from build123d import *

# Parameters (mm, degrees)
SKETCH1_R                 = 4.7625
BOSS_EXTRUDE1_DEPTH       = 6.604
CUT_EXTRUDE1_DEPTH        = 7.604
SKETCH3_W                 = 6.604
SKETCH3_H                 = 6.35
BOSS_EXTRUDE2_DEPTH       = 6.604
FILLET1_R                 = 6.35
FILLET2_R                 = 3.175
F_4_40_TAPPED_HOLE1_D     = 2.2606
F_4_40_TAPPED_HOLE1_DEPTH = 7.5946
F_4_40_TAPPED_HOLE1_TIP   = 0.679152758


with BuildPart() as part:
    # Sketch1 → Boss-Extrude1 (new body)
    with BuildSketch(Plane.XY):
        Polygon((0, 0), (0, 69.85), (-19.939, 69.85), (-19.939, 50.8), (-25.4, 45.339), (-25.4, 0), align=None)
        with Locations((-9.9695, 57.15)):
            Circle(SKETCH1_R, mode=Mode.SUBTRACT)
    extrude(amount=BOSS_EXTRUDE1_DEPTH)

    # Sketch2 → Cut-Extrude1 (cut, through all)
    with BuildSketch(Plane.XY.offset(6.604)):
        Polygon((-12.2936, 37.0078), (-13.716, 37.0078), (-13.716, 32.8422), (-12.2936, 32.8422), (-12.2936, 30.5562), (-6.35, 30.5562), (-6.35, 32.8422), (0, 32.8422), (0, 37.0078), (-6.35, 37.0078), (-6.35, 39.2938), (-12.2936, 39.2938), align=None)
        Polygon((-12.2936, 20.2438), (-12.2936, 17.9578), (-13.716, 17.9578), (-13.716, 13.7922), (-12.2936, 13.7922), (-12.2936, 11.5062), (-6.35, 11.5062), (-6.35, 13.7922), (0, 13.7922), (0, 17.9578), (-6.35, 17.9578), (-6.35, 20.2438), align=None)
    extrude(amount=-CUT_EXTRUDE1_DEPTH, mode=Mode.SUBTRACT)

    # Sketch3 → Boss-Extrude2 (add)
    with BuildSketch(Plane.XY.offset(6.604)):
        with Locations((3.302, 44.45)):
            Rectangle(SKETCH3_W, SKETCH3_H)
        with Locations((3.302, 25.4)):
            Rectangle(SKETCH3_W, SKETCH3_H)
        with Locations((3.302, 6.35)):
            Rectangle(SKETCH3_W, SKETCH3_H)
    extrude(amount=-BOSS_EXTRUDE2_DEPTH)

    # Fillet1
    fillet1_edges = [part.edges().sort_by_distance(p)[0] for p in [
        (-25.4, 0, 3.302),
        (-25.4, 45.339, 3.302),
        (-19.939, 50.8, 3.302),
        (0, 69.85, 3.302),
    ]]
    fillet(fillet1_edges, radius=FILLET1_R)

    # Fillet2
    fillet2_edges = [part.edges().sort_by_distance(p)[0] for p in [
        (-19.939, 69.85, 3.302),
    ]]
    fillet(fillet2_edges, radius=FILLET2_R)

    # #4-40 Tapped Hole1
    with Locations(Plane.XY.offset(6.604)):
        with Locations((-3.6195, 49.53), (-16.3195, 49.53)):
            Hole(F_4_40_TAPPED_HOLE1_D / 2, depth=F_4_40_TAPPED_HOLE1_DEPTH)
            with Locations((0, 0, -(F_4_40_TAPPED_HOLE1_DEPTH + F_4_40_TAPPED_HOLE1_TIP / 2))):  # 118° drill point
                Cone(0, F_4_40_TAPPED_HOLE1_D / 2, F_4_40_TAPPED_HOLE1_TIP, mode=Mode.SUBTRACT)


solid = part.part
For this review, take the finished solid that the model builds, in its own axes (mm). A direction names the side the tool comes from. Give positions to 0.01 mm unless a question says otherwise; leave off trailing zeros. Order: outer loops, then holes, each group sorted by start corner. A loop starts at its lowest first (then second) coordinate and runs counter-clockwise, first axis right, second up. Notation, with made-up numbers: M 48.25,-36.75 L 98.25,-36.75 A19 cw 98.25,-31.75 Z; hole C -5.75,81 d2. An arc over 180 degrees is marked long. Answer in a Markdown table with one row per item. Add a question column.
(1) For pin 1 (4 mm diameter, centred on x = -8, y = 7, fed in from -Z); pin 2 (1.1 mm diameter, centred on y = 12.5, z = 2, fed in from +X); pin 3 (3.5 mm diameter, centred on x = 3.5, z = 4, fed in from +Y) (3 decimals); pin 4 (2 mm diameter, centred on x = -10, y = 55, fed in from +Z), all flat-tipped, find the tip position at first contact; note any pin that passes through.
(2) Mouldability with a two-part tool opening along Y and no side actions: class faces 1 (the face through (-3, 32.842, 3)), 2 (the face through (6.604, 6, 3)), 3 (the face through (-1.91, 68.04, 3.35)) as +Y half, -Y half, draft (parallel to the pull), parting line (faces both ways), or undercut.
(3) Consider section B-B on x = -8. State the section outline as (y, z) points, and give its area (3 significant figures).
(4) Consider section A-A on y = 57.15. State the section outline as (x, z) points, and give its area (3 significant figures).
(5) Consider section C-C on z = 0.75. Give the number of separate pieces and of enclosed holes in the cut face, and give its area (3 significant figures).
(6) Wall thickness on probe 1 along Y at (x, z) = (-6.5, 6.25); probe 2 along Y at (x, z) = (-7, 4); probe 3 along X at (y, z) = (18, 4.5): over which ranges is each line inside the solid? List them lowest first. Write a range as [from, to].
(7) For faces 4 (the face through (0, 2, 3)), 5 (the face through (-9, 11.506, 3)), 6 (the face through (-13, 17.958, 3)), list the 3-axis set-ups (+Z, -Z, +X, -X, +Y, -Y) from which the entire face can be reached by the end or side of a thin tool; tool diameter is ignored.
Evaluation:
| question | item | result |
|---|---|---|
| 1 | pin 1 | stops at z = 0 |
| 1 | pin 2 | stops at x = 0 |
| 1 | pin 3 | stops at y = 47.625 |
| 1 | pin 4 | passes through |
| 2 | face 1 | undercut |
| 2 | face 2 | draft |
| 2 | face 3 | +Y half |
| 3 | outline | M 0,0 L 11.51,0 L 11.51,6.6 L 0,6.6 Z; M 20.24,0 L 30.56,0 L 30.56,6.6 L 20.24,6.6 Z; M 39.29,0 L 52.81,0 L 52.81,6.6 L 39.29,6.6 Z; M 61.49,0 L 69.85,0 L 69.85,6.6 L 61.49,6.6 Z |
| 3 | area | 289 mm^2 |
| 4 | outline | M -19.94,0 L -14.73,0 L -14.73,6.6 L -19.94,6.6 Z; M -5.21,0 L 0,0 L 0,6.6 L -5.21,6.6 Z |
| 4 | area | 68.8 mm^2 |
| 5 | separate pieces | 1 |
| 5 | enclosed holes | 3 |
| 5 | area | 1,510 mm^2 |
| 6 | probe 1 | y = [0, 11.51], [20.24, 30.56], [39.29, 53.89], [60.41, 69.85] |
| 6 | probe 2 | y = [0, 11.51], [20.24, 30.56], [39.29, 53.43], [60.87, 69.85] |
| 6 | probe 3 | x = [-25.4, -12.29], [-6.35, 0] |
| 7 | face 4 | +Z, -Z, +X, -Y |
| 7 | face 5 | +Z, -Z |
| 7 | face 6 | +Z, -Z, +X |
